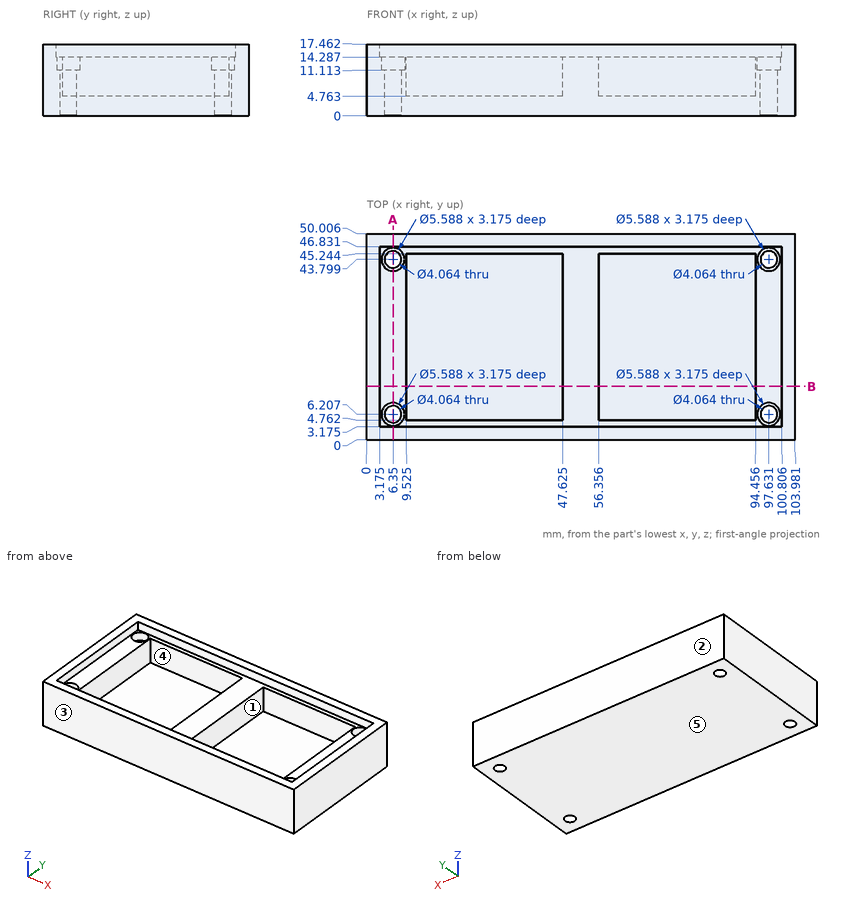
Part print with two shaded views. Sizes in mm from the minimum x, y, z corner. A direction names the side the tool comes from. Give positions to 0.01 mm unless a question says otherwise; leave off trailing zeros. Order: outer loops, then holes, each group sorted by start corner. A loop starts at its lowest first (then second) coordinate and runs counter-clockwise, first axis right, second up.
1) 3-axis set-ups, long thin cutter, end or side, ignore diameter. For the marked faces 4 and 5: which of +Z, -Z, +X, -X, +Y, -Y reach the whole face in a straight line?
2) Wall check: probe 1 along X at (y, z) = (32.5, 9) (1 decimal); probe 2 along Y at (x, z) = (6.35, 4.25) (1 decimal); probe 3 along Y at (x, z) = (85, 5.5). Give the ranges that are in metal, low to high.
3) Pin check, flat tips, straight feed: pin 1 (3 mm diameter, centred on y = 29, z = 8, fed in from -X); pin 2 (3 mm diameter, centred on x = 5, y = 45, fed in from +Z); pin 3 (22 mm diameter, centred on x = 30, y = 16.5, fed in from +Z); pin 4 (4.5 mm diameter, centred on x = 97.63, y = 43.8, fed in from +Z). Stop position of each tip, or through.
4) Saw through at A-A, the plane x = 6.35. Count the separate pieces of the cut face and the enclosed holes in it, then the cut area to 3 significant figures.
5) Saw through at B-B, the plane y = 13. Write the cut outline in (x, z) (1 decimal).
6) Mould opens along Y. For the marked faces 1, 2 and 3 say: +Y half, -Y half, draft (parallel to the pull), parting line (faces both ways), or undercut.
Computed:
1. face 4: +Z
1. face 5: -Z, +X, -X, +Y, -Y
2. probe 1: x = 0 to 9.5, 47.6 to 56.4, 94.5 to 104
2. probe 2: y = 0 to 4.2, 8.2 to 41.8, 45.8 to 50
2. probe 3: y = 0 to 4.76, 45.24 to 50.01
3. pin 1: stops at x = 0
3. pin 2: stops at z = 14.29
3. pin 3: stops at z = 4.76
3. pin 4: stops at z = 11.11
4. separate pieces: 3
4. enclosed holes: 0
4. area: 609 mm2
5. outline: (0, 0) - (104, 0) - (104, 17.5) - (100.8, 17.5) - (100.8, 14.3) - (94.5, 14.3) - (94.5, 4.8) - (56.4, 4.8) - (56.4, 14.3) - (47.6, 14.3) - (47.6, 4.8) - (9.5, 4.8) - (9.5, 14.3) - (3.2, 14.3) - (3.2, 17.5) - (0, 17.5) - close
6. face 1: undercut
6. face 2: +Y half
6. face 3: -Y half
